Read the model definition and answer for the solid it produces. Units are mm, in the model's axes. A direction names the side the tool comes from. Coordinates: 2 decimals unless noted, no trailing zeros. Loops run counter-clockwise (first coordinate to the right, second up) from the corner with the lowest first, then second, coordinate; pieces in that order, holes last. Notation, with made-up numbers: (-32.5, 81.25) -> (24.5, 81.25) arc R29 ccw to (24.5, 112.25) -> close; hole circle Ø3 at (66.5, 5). An arc over 180 degrees is marked (long way). Answer as a JSON object with one key per item and string values. Group by question number.
Q1. Straight lines are drawn through the part: line 1 along Y through (x, z) = (5, 1.65); line 2 along Y through (x, z) = (73, 0.6); line 3 along X through (y, z) = (25, 1.8). For each, find the intervals that lie inside material, in ascending order. Write a range as [from, to].
Q2. Determine the mould class of faces 1 (the cylindrical face through (2, 39, 1)), 2 (the flat face through (56.404, 25, 1)), 3 (the flat face through (83, 8.722, 1)), 4 (the flat face through (100, 20, 1)) for opening direction Y: released by +Y, released by -Y, zero draft, split by the parting line, or undercut.
Q3. This flat-tipped pin is pushed along its axis until it touches: P1, Ø1, axis at x = 58, y = 20.5, coming from the -Z side. Where does it stop, or does it pass through?
Q4. The part is cut by section A-A on x = 14.5. Write down the section's boundary in (y, z), and give its area (3 significant figures).
Q5. For faces 5 (the flat face through (84.061, 14, 1)), 6 (the flat face through (49, 20, 0)), determine the directions among +Z, -Z, +X, -X, +Y, -Y from which every point of the face is accessible in a straight line to the end or side of a thin tool.
Q6. The part is cut by section B-B on x = 75. State how many separate pieces and enclosed holes the cut face has, and give its area (3 significant figures).
from build123d import *

# Parameters (mm, degrees)
F0_W     = 4.3279479289
F0_H     = 15.8676286083
F0_R     = 2
F1_DEPTH = 2


with BuildPart() as f1:
    # F0 (on Top) → F1 (new body)
    with BuildSketch(Plane.XY):
        with BuildLine():
            ThreePointArc((0, 5), (1.4644660941, 1.4644660941), (5, 0))
            Line((5, 0), (95, 0))
            ThreePointArc((95, 0), (98.5355339059, 1.4644660941), (100, 5))
            Line((100, 5), (100, 35))
            ThreePointArc((100, 35), (98.5355339059, 38.5355339059), (95, 40))
            Line((95, 40), (5, 40))
            ThreePointArc((5, 40), (1.4644660941, 38.5355339059), (0, 35))
            Line((0, 35), (0, 5))
        make_face()
        Polygon((20.4271134466, 8.7217205013), (7.6113012163, 8.7217205013), (7.6113012163, 29.4713470357), (12.0119114399, 29.4713470357), (12.0119114399, 12.3548352371), (20.4271134466, 12.3548352371), align=None, mode=Mode.SUBTRACT)
        with Locations((25.8563492798, 16.6555348055)):
            Rectangle(F0_W, F0_H, mode=Mode.SUBTRACT)
        with BuildLine():
            Line((47.2077104423, 19.0670147113), (47.2077104423, 8.7217205013))
            Line((47.2077104423, 8.7217205013), (42.8797625133, 8.7217205013))
            Line((42.8797625133, 8.7217205013), (42.8797625133, 17.9907044709))
            add(Edge.make_bspline(
                [(42.8797625133, 17.9907044709), (42.8797625133, 19.7073511835), (42.2689450984, 20.5656745398)],
                knots=[0, 0, 0, 1, 1, 1], degree=2))
            add(Edge.make_bspline(
                [(42.2689450984, 20.5656745398), (41.6581276834, 21.4239978961), (40.3229580181, 21.4239978961)],
                knots=[0, 0, 0, 1, 1, 1], degree=2))
            add(Edge.make_bspline(
                [(40.3229580181, 21.4239978961), (38.5064006502, 21.4239978961), (37.6980326215, 20.2114458531)],
                knots=[0, 0, 0, 1, 1, 1], degree=2))
            add(Edge.make_bspline(
                [(37.6980326215, 20.2114458531), (36.8896645928, 18.99889381), (36.8896645928, 16.1877712833)],
                knots=[0, 0, 0, 1, 1, 1], degree=2))
            Line((36.8896645928, 16.1877712833), (36.8896645928, 8.7217205013))
            Line((36.8896645928, 8.7217205013), (32.5617166639, 8.7217205013))
            Line((32.5617166639, 8.7217205013), (32.5617166639, 24.5893491096))
            Line((32.5617166639, 24.5893491096), (35.8678510734, 24.5893491096))
            Line((35.8678510734, 24.5893491096), (36.4491494311, 22.559346251))
            Line((36.4491494311, 22.559346251), (36.6898432823, 22.559346251))
            add(Edge.make_bspline(
                [(36.6898432823, 22.559346251), (37.4164662295, 23.7083187862), (38.6857856903, 24.296429234)],
                knots=[0, 0, 0, 1, 1, 1], degree=2))
            add(Edge.make_bspline(
                [(38.6857856903, 24.296429234), (39.9551051511, 24.8845396819), (41.5718412085, 24.8845396819)],
                knots=[0, 0, 0, 1, 1, 1], degree=2))
            add(Edge.make_bspline(
                [(41.5718412085, 24.8845396819), (44.3420911945, 24.8845396819), (45.7749008184, 23.3881505501)],
                knots=[0, 0, 0, 1, 1, 1], degree=2))
            add(Edge.make_bspline(
                [(45.7749008184, 23.3881505501), (47.2077104423, 21.8917614183), (47.2077104423, 19.0670147113)],
                knots=[0, 0, 0, 1, 1, 1], degree=2))
        make_face(mode=Mode.SUBTRACT)
        Polygon((61.3995648787, 20.2886495412), (68.6930427106, 8.7217205013), (63.697509949, 8.7217205013), (58.2614620257, 17.4639028342), (56.4040321171, 16.1287331688), (56.4040321171, 8.7217205013), (52.0034218934, 8.7217205013), (52.0034218934, 29.4713470357), (56.4040321171, 29.4713470357), (56.4040321171, 19.9752933952), (58.1343030099, 22.418563055), (63.7565480635, 29.4713470357), (68.6385459896, 29.4713470357), align=None, mode=Mode.SUBTRACT)
        with BuildLine():
            Line((84.0611180428, 8.7217205013), (81.0410914187, 8.7217205013))
            Line((81.0410914187, 8.7217205013), (80.200933636, 10.8788823757))
            Line((80.200933636, 10.8788823757), (80.0873988006, 10.8788823757))
            add(Edge.make_bspline(
                [(80.0873988006, 10.8788823757), (78.9974643798, 9.5028401695), (77.8394090578, 8.9692264427)],
                knots=[0, 0, 0, 1, 1, 1], degree=2))
            add(Edge.make_bspline(
                [(77.8394090578, 8.9692264427), (76.6813537358, 8.4356127159), (74.8239238272, 8.4356127159)],
                knots=[0, 0, 0, 1, 1, 1], degree=2))
            add(Edge.make_bspline(
                [(74.8239238272, 8.4356127159), (72.5396029371, 8.4356127159), (71.2271402388, 9.7435340208)],
                knots=[0, 0, 0, 1, 1, 1], degree=2))
            add(Edge.make_bspline(
                [(71.2271402388, 9.7435340208), (69.9146775405, 11.0514553256), (69.9146775405, 13.4629352315)],
                knots=[0, 0, 0, 1, 1, 1], degree=2))
            add(Edge.make_bspline(
                [(69.9146775405, 13.4629352315), (69.9146775405, 15.9879499728), (71.6812795808, 17.1868778356)],
                knots=[0, 0, 0, 1, 1, 1], degree=2))
            add(Edge.make_bspline(
                [(71.6812795808, 17.1868778356), (73.447881621, 18.3858056984), (77.008334062, 18.5129647141)],
                knots=[0, 0, 0, 1, 1, 1], degree=2))
            Line((77.008334062, 18.5129647141), (79.7649598678, 18.5992511891))
            Line((79.7649598678, 18.5992511891), (79.7649598678, 19.2940843823))
            add(Edge.make_bspline(
                [(79.7649598678, 19.2940843823), (79.7649598678, 21.7055642881), (77.2944418475, 21.7055642881)],
                knots=[0, 0, 0, 1, 1, 1], degree=2))
            add(Edge.make_bspline(
                [(77.2944418475, 21.7055642881), (75.3915980046, 21.7055642881), (72.8211693291, 20.556591753)],
                knots=[0, 0, 0, 1, 1, 1], degree=2))
            Line((72.8211693291, 20.556591753), (71.3906304019, 23.4812491152))
            add(Edge.make_bspline(
                [(71.3906304019, 23.4812491152), (74.129090634, 24.9163294358), (77.462473404, 24.9163294358)],
                knots=[0, 0, 0, 1, 1, 1], degree=2))
            add(Edge.make_bspline(
                [(77.462473404, 24.9163294358), (80.655072978, 24.9163294358), (82.3580955104, 23.5243923527)],
                knots=[0, 0, 0, 1, 1, 1], degree=2))
            add(Edge.make_bspline(
                [(82.3580955104, 23.5243923527), (84.0611180428, 22.1324552696), (84.0611180428, 19.2940843823)],
                knots=[0, 0, 0, 1, 1, 1], degree=2))
            Line((84.0611180428, 19.2940843823), (84.0611180428, 8.7217205013))
        make_face(mode=Mode.SUBTRACT)
        with Locations((90.6847403453, 16.6555348055)):
            Rectangle(F0_W, F0_H, mode=Mode.SUBTRACT)
        with BuildLine():
            add(Edge.make_bspline(
                [(25.8631613699, 26.5603138537), (23.5061781851, 26.5603138537), (23.5061781851, 28.6902273676)],
                knots=[0, 0, 0, 1, 1, 1], degree=2))
            add(Edge.make_bspline(
                [(23.5061781851, 28.6902273676), (23.5061781851, 30.8065167011), (25.8631613699, 30.8065167011)],
                knots=[0, 0, 0, 1, 1, 1], degree=2))
            add(Edge.make_bspline(
                [(25.8631613699, 30.8065167011), (28.2201445547, 30.8065167011), (28.2201445547, 28.6902273676)],
                knots=[0, 0, 0, 1, 1, 1], degree=2))
            add(Edge.make_bspline(
                [(28.2201445547, 28.6902273676), (28.2201445547, 27.6820380284), (27.6320341068, 27.1211759411)],
                knots=[0, 0, 0, 1, 1, 1], degree=2))
            add(Edge.make_bspline(
                [(27.6320341068, 27.1211759411), (27.043923659, 26.5603138537), (25.8631613699, 26.5603138537)],
                knots=[0, 0, 0, 1, 1, 1], degree=2))
        make_face(mode=Mode.SUBTRACT)
        with Locations((5, 35)):
            Circle(F0_R, mode=Mode.SUBTRACT)
        with BuildLine():
            add(Edge.make_bspline(
                [(90.6915524354, 26.5603138537), (88.3345692506, 26.5603138537), (88.3345692506, 28.6902273676)],
                knots=[0, 0, 0, 1, 1, 1], degree=2))
            add(Edge.make_bspline(
                [(88.3345692506, 28.6902273676), (88.3345692506, 30.8065167011), (90.6915524354, 30.8065167011)],
                knots=[0, 0, 0, 1, 1, 1], degree=2))
            add(Edge.make_bspline(
                [(90.6915524354, 30.8065167011), (93.0485356202, 30.8065167011), (93.0485356202, 28.6902273676)],
                knots=[0, 0, 0, 1, 1, 1], degree=2))
            add(Edge.make_bspline(
                [(93.0485356202, 28.6902273676), (93.0485356202, 27.6820380284), (92.4604251724, 27.1211759411)],
                knots=[0, 0, 0, 1, 1, 1], degree=2))
            add(Edge.make_bspline(
                [(92.4604251724, 27.1211759411), (91.8723147246, 26.5603138537), (90.6915524354, 26.5603138537)],
                knots=[0, 0, 0, 1, 1, 1], degree=2))
        make_face(mode=Mode.SUBTRACT)
    extrude(amount=F1_DEPTH)


solid = f1.part
Final values:
{
 "1": {"line 1": "y = [0, 33], [37, 40]", "line 2": "y = [0, 8.69], [17.85, 20.64], [24.18, 40]", "line 3": "x = [0, 7.61], [12.01, 52], [56.4, 60.19], [65.11, 100]"},
 "2": {"face 1": "released by +Y", "face 2": "undercut", "face 3": "undercut", "face 4": "zero draft"},
 "3": {"P1": "passes through"},
 "4": {"outline": "(0, 0) -> (8.72, 0) -> (8.72, 2) -> (0, 2) -> close; (12.35, 0) -> (40, 0) -> (40, 2) -> (12.35, 2) -> close", "area": "72.7 mm2"},
 "5": {"face 5": "+Z, -Z", "face 6": "-Z, +X, -X, +Y, -Y"},
 "6": {"separate pieces": "3", "enclosed holes": "0", "area": "53.5 mm2"}
}
